Input: part model. Units: mm. Frame: model coordinates. A direction names the side the tool comes from. Give positions to 0.01 mm unless a question says otherwise; leave off trailing zeros. Loops run counter-clockwise (first coordinate to the right, second up) from the corner with the lowest first, then second, coordinate; pieces in that order, holes last. Notation, with made-up numbers: M -18.75,75 L -8.75,75 A20 ccw -8.75,79 Z; hole C 12,-2 d8. An arc over 180 degrees is marked long. Use CSV: the item, a comma, the result in double quotes. Start each with the question number.
Q1. Reachability of faces 4 (the cylindrical face through (11.43, 11.196, 0.459)), 5 (the cylindrical face through (-11.43, -11.196, 25.212)), 6 (the flat face through (-13.1, 8.4, 22.5)), 7 (the cylindrical face through (11.196, -11.43, 0.459)) from +Z, -Z, +X, -X, +Y, -Y: full face, straight path, thin tool, end or side. Return the list, or none.
Q2. Pin query (flat end, axial travel): pin 1 (1.5 mm diameter, centred on x = 7.5, z = 0.5, fed in from -Y); pin 2 (5 mm diameter, centred on y = -1.5, z = -7.5, fed in from +X); pin 3 (10 mm diameter, centred on y = 14, z = 7.5, fed in from +X); pin 4 (8 mm diameter, centred on x = 7.5, y = -9.5, fed in from -Z). Return the tip coordinate at first contact, or that it passes through.
Q3. Pull-direction query (X, two-part tool) for faces 1 (the cylindrical face through (11.43, 11.196, 25.212)), 2 (the flat face through (4.6, -15.5, 28)), 3 (the flat face through (2.7, -8.5, 20)); classes: released by +X, released by -X, zero draft, split by the parting line, or undercut.
Q4. Section A-A, the plane z = -4. Output: boundary loops of the cut face in (x, y), plus the area to 3 significant figures.
Q5. Section B-B, the plane y = -17. Output: boundary loops of the cut face in (x, z), plus the area to 3 significant figures.
Q6. Section D-D, the plane x = 0. State how many separate pieces and enclosed holes the cut face has, plus the area to 3 significant figures.
Q7. Material intervals for line 1 along Y through (x, z) = (0, 28.75); line 2 along Z through (x, y) = (16, -7); line 3 along Z through (x, y) = (-10.5, 7), sorted ascending.
from build123d import *

# Parameters (mm, degrees)
HOLLOW_HUB_START               = -20
SKETCH_1_R                     = 16
SKETCH_1_R_2                   = 8.7
HOLLOW_HUB_DEPTH               = 48
REAR_STACK_FLANGE_START        = -21.5
SKETCH_2_R                     = 22.2
SKETCH_2_R_2                   = 13
REAR_STACK_FLANGE_DEPTH        = 1.5
SUN_MOUNT_FLANGE_START         = 28
SKETCH_3_R                     = 21
SKETCH_3_R_2                   = 8.7
SUN_MOUNT_FLANGE_DEPTH         = 4
REAR_ROTOR_BEARING_SEAT_START  = -20
SKETCH_4_R                     = 13
REAR_ROTOR_BEARING_SEAT_DEPTH  = 5
FRONT_ROTOR_BEARING_SEAT_START = 15
SKETCH_5_R                     = 13
FRONT_ROTOR_BEARING_SEAT_DEPTH = 5
CIRCLIP_GROOVE_START           = 21.5
SKETCH_6_R                     = 17
SKETCH_6_R_2                   = 15.4
CIRCLIP_GROOVE_DEPTH           = 1
SKETCH_7_R                     = 1.25
THROUGH_HOLES_DEPTH            = 100


with BuildPart() as part:
    # Эскиз1 → Hollow_hub (new body)
    with BuildSketch(Plane.XY.offset(HOLLOW_HUB_START)):
        Circle(SKETCH_1_R)
        Circle(SKETCH_1_R_2, mode=Mode.SUBTRACT)
    extrude(amount=HOLLOW_HUB_DEPTH)

    # Эскиз2 → Rear_stack_flange (add)
    with BuildSketch(Plane.XY.offset(REAR_STACK_FLANGE_START)):
        Circle(SKETCH_2_R)
        Circle(SKETCH_2_R_2, mode=Mode.SUBTRACT)
    extrude(amount=REAR_STACK_FLANGE_DEPTH)

    # Эскиз3 → Sun_mount_flange (add)
    with BuildSketch(Plane.XY.offset(SUN_MOUNT_FLANGE_START)):
        Circle(SKETCH_3_R)
        Circle(SKETCH_3_R_2, mode=Mode.SUBTRACT)
    extrude(amount=SUN_MOUNT_FLANGE_DEPTH)

    # Эскиз4 → Rear_rotor_bearing_seat (cut)
    with BuildSketch(Plane.XY.offset(REAR_ROTOR_BEARING_SEAT_START)):
        Circle(SKETCH_4_R)
    extrude(amount=REAR_ROTOR_BEARING_SEAT_DEPTH, mode=Mode.SUBTRACT)

    # Эскиз5 → Front_rotor_bearing_seat (cut)
    with BuildSketch(Plane.XY.offset(FRONT_ROTOR_BEARING_SEAT_START)):
        Circle(SKETCH_5_R)
    extrude(amount=FRONT_ROTOR_BEARING_SEAT_DEPTH, mode=Mode.SUBTRACT)

    # Эскиз6 → Circlip_groove (cut)
    with BuildSketch(Plane.XY.offset(CIRCLIP_GROOVE_START)):
        Circle(SKETCH_6_R)
        Circle(SKETCH_6_R_2, mode=Mode.SUBTRACT)
    extrude(amount=CIRCLIP_GROOVE_DEPTH, mode=Mode.SUBTRACT)

    # Эскиз7 → Through_holes (cut, symmetric)
    with BuildSketch(Plane.XY):
        with Locations((17, 0)):
            Circle(SKETCH_7_R)
        with Locations((0, 17)):
            Circle(SKETCH_7_R)
        with Locations((-17, 0)):
            Circle(SKETCH_7_R)
        with Locations((0, -17)):
            Circle(SKETCH_7_R)
    extrude(amount=THROUGH_HOLES_DEPTH, both=True, mode=Mode.SUBTRACT)


solid = part.part
A:
1,face 4,"+X, +Y"
1,face 5,"-X, -Y"
1,face 6,"none"
1,face 7,"+X, -Y"
2,pin 1,"y = -14.51"
2,pin 2,"x = 15.98"
2,pin 3,"x = 13.23"
2,pin 4,"z = -21.5"
3,face 1,"released by +X"
3,face 2,"zero draft"
3,face 3,"undercut"
4,outline,"M -15.98,-0.73 A16 ccw -0.73,-15.98 A1.25 cw 0.73,-15.98 A16 ccw 15.98,-0.73 A1.25 cw 15.98,0.73 A16 ccw 0.73,15.98 A1.25 cw -0.73,15.98 A16 ccw -15.98,0.73 A1.25 cw Z; hole C 0,0 d17.4"
4,area,"565 mm^2"
5,outline,"M -14.28,-21.5 L -1.25,-21.5 L -1.25,-20 L -14.28,-20 Z; M -12.33,28 L -1.25,28 L -1.25,32 L -12.33,32 Z; M 1.25,-21.5 L 14.28,-21.5 L 14.28,-20 L 1.25,-20 Z; M 1.25,28 L 12.33,28 L 12.33,32 L 1.25,32 Z"
5,area,"128 mm^2"
6,separate pieces,"6"
6,enclosed holes,"0"
6,area,"689 mm^2"
7,line 1,"-21 to -18.25, -15.75 to -8.7, 8.7 to 15.75, 18.25 to 21"
7,line 2,"-21.5 to -20, 28 to 32"
7,line 3,"-15 to 15, 20 to 32"
